Could you check a few things on this model? Use its own coordinates, in mm. Face numbers are marked on the shaded views. A direction names the side the tool comes from. Coordinates: 2 decimals unless noted, no trailing zeros. Loops run counter-clockwise (first coordinate to the right, second up) from the corner with the lowest first, then second, coordinate; pieces in that order, holes last.
1) If I drill on line 1 along Y through (x, z) = (51.65, 24.1); line 2 along X through (y, z) = (0.2, 13.5); line 3 along Z through (x, y) = (21.5, 35), over which ranges is the centre line in solid material (lowest first)?
2) Imagine slicing it at B-B on y = 40.25. Please give me the cut outline in (x, z), plus the area to 3 significant figures.
3) Imagine slicing it at D-D on x = 51.65. Please give me the cut outline in (y, z).
4) Imagine slicing it at C-C on z = 13.5. Please give me the cut outline in (x, y), plus the area to 3 significant figures.
5) Will these pins go through, and if not, where does the flat tip stop? P1, Ø3, axis at x = 20.65, y = 40.25, coming from the +Z side (3 decimals); P2, Ø3, axis at y = 34, z = 22, coming from the -X side; P3, Ø9, axis at x = 64.8, z = 13.5, coming from the +Y side; P4, Ø5.5, axis at x = 51.65, y = 9.25, coming from the -Z side.
6) For the marked faces 1 and 2, which set-ups out of +Z, -Z, +X, -X, +Y, -Y let a thin tool reach every point of the face, with its end or its side?
7) Imagine slicing it at A-A on x = 7.5. Please give me the cut outline in (y, z).
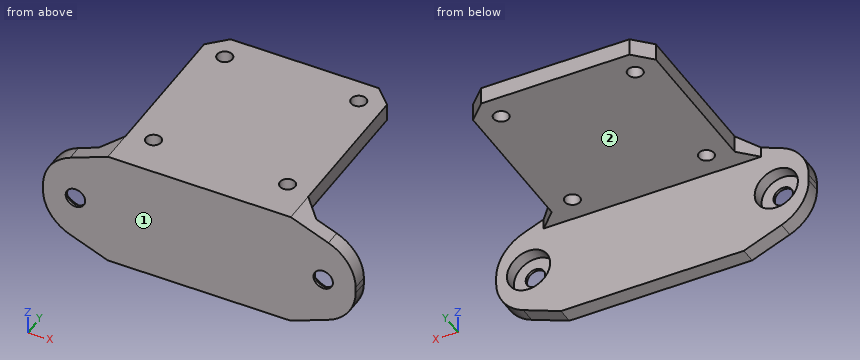
```python
from build123d import *

# Parameters (mm, degrees)
SCHIZZO2_W                                           = 72.3
SCHIZZO2_H                                           = 27
ESTRUSIONE_ESTRUSIONE1_DEPTH                         = 3.6
SCHIZZO3_W                                           = 42.3
SCHIZZO3_H                                           = 4
ESTRUSIONE_ESTRUSIONE2_DEPTH                         = 42.3
SCHIZZO4_R                                           = 1.75
TAGLIO_ESTRUSIONE1_DEPTH                             = 42.3
FORO_LAMATO_PER_VITE_M4_A_TESTA_CILINDRI_D           = 4.5
FORO_LAMATO_PER_VITE_M4_A_TESTA_CILINDRI_DEPTH       = 9
FORO_LAMATO_PER_VITE_M4_A_TESTA_CILINDRI_CBORE_D     = 10
FORO_LAMATO_PER_VITE_M4_A_TESTA_CILINDRI_CBORE_DEPTH = 3
FORO_LAMATO_PER_VITE_M4_A_TESTA_CILINDRI_TIP         = 1.351936393
TAGLIO_ESTRUSIONE2_DEPTH                             = 42.3
SMUSSO1_SIZE                                         = 4
RACCORDO1_R                                          = 10
SMUSSO2_SIZE                                         = 4


with BuildPart() as part:
    # Schizzo2 → Estrusione-Estrusione1 (new body)
    with BuildSketch(Plane(origin=(0, 0, 0), x_dir=(1, 0, 0), z_dir=(0, 1, 0))):
        with Locations((36.15, -13.5)):
            Rectangle(SCHIZZO2_W, SCHIZZO2_H)
    extrude(amount=ESTRUSIONE_ESTRUSIONE1_DEPTH)

    # Schizzo3 → Estrusione-Estrusione2 (add)
    with BuildSketch(Plane(origin=(0, 3.6, 0), x_dir=(1, 0, 0), z_dir=(0, 1, 0))):
        with Locations((36.15, -25)):
            Rectangle(SCHIZZO3_W, SCHIZZO3_H)
    extrude(amount=ESTRUSIONE_ESTRUSIONE2_DEPTH)

    # Schizzo4 → Taglio-Estrusione1 (cut)
    with BuildSketch(Plane.XY.offset(27)):
        with Locations((20.65, 40.25)):
            Circle(SCHIZZO4_R)
        with Locations((51.65, 40.25)):
            Circle(SCHIZZO4_R)
        with Locations((51.65, 9.25)):
            Circle(SCHIZZO4_R)
        with Locations((20.65, 9.25)):
            Circle(SCHIZZO4_R)
    extrude(amount=-TAGLIO_ESTRUSIONE1_DEPTH, mode=Mode.SUBTRACT)

    # Foro lamato per Vite M4 a testa cilindrica-2
    with Locations(Plane(origin=(0, 3.6, 0), x_dir=(1, 0, 0), z_dir=(0, 1, 0))):
        with Locations((7.5, -13.5), (64.8, -13.5)):
            CounterBoreHole(FORO_LAMATO_PER_VITE_M4_A_TESTA_CILINDRI_D / 2, FORO_LAMATO_PER_VITE_M4_A_TESTA_CILINDRI_CBORE_D / 2, FORO_LAMATO_PER_VITE_M4_A_TESTA_CILINDRI_CBORE_DEPTH, depth=FORO_LAMATO_PER_VITE_M4_A_TESTA_CILINDRI_DEPTH)
            with Locations((0, 0, -(FORO_LAMATO_PER_VITE_M4_A_TESTA_CILINDRI_DEPTH + FORO_LAMATO_PER_VITE_M4_A_TESTA_CILINDRI_TIP / 2))):  # 118° drill point
                Cone(0, FORO_LAMATO_PER_VITE_M4_A_TESTA_CILINDRI_D / 2, FORO_LAMATO_PER_VITE_M4_A_TESTA_CILINDRI_TIP, mode=Mode.SUBTRACT)

    # Schizzo8 → Taglio-Estrusione2 (cut)
    with BuildSketch(Plane(origin=(0, 3.6, 0), x_dir=(1, 0, 0), z_dir=(0, 1, 0))):
        Polygon((15, -27), (0, -21), (0, -27), align=None)
        Polygon((0, -6), (0, 0), (15, 0), align=None)
        Polygon((57.3, 0), (72.3, 0), (72.3, -6), align=None)
        Polygon((57.3, -27), (72.3, -27), (72.3, -21), align=None)
    extrude(amount=-TAGLIO_ESTRUSIONE2_DEPTH, mode=Mode.SUBTRACT)

    # Smusso1
    smusso1_edges = [part.edges().sort_by_distance(p)[0] for p in [
        (15, 45.9, 25),
        (57.3, 45.9, 25),
    ]]
    chamfer(smusso1_edges, length=SMUSSO1_SIZE)

    # Raccordo1
    raccordo1_edges = [part.edges().sort_by_distance(p)[0] for p in [
        (0, 1.8, 21),
        (72.3, 1.8, 21),
        (72.3, 1.8, 6),
        (0, 1.8, 6),
    ]]
    fillet(raccordo1_edges, radius=RACCORDO1_R)

    # Smusso2
    smusso2_edges = [part.edges().sort_by_distance(p)[0] for p in [
        (15, 3.6, 25),
        (57.3, 3.6, 25),
    ]]
    chamfer(smusso2_edges, length=SMUSSO2_SIZE)


solid = part.part
```
Filled in:
1. line 1: y = 0 to 7.5, 11 to 38.5, 42 to 45.9
1. line 2: x = 0 to 5.25, 9.75 to 62.55, 67.05 to 72.3
1. line 3: z = 23 to 27
2. outline: (15, 23) - (18.9, 23) - (18.9, 27) - (15, 27) - close; (22.4, 23) - (49.9, 23) - (49.9, 27) - (22.4, 27) - close; (53.4, 23) - (57.3, 23) - (57.3, 27) - (53.4, 27) - close
2. area: 141 mm2
3. outline: (0, 0) - (3.6, 0) - (3.6, 23) - (7.5, 23) - (7.5, 27) - (0, 27) - close; (11, 23) - (38.5, 23) - (38.5, 27) - (11, 27) - close; (42, 23) - (45.9, 23) - (45.9, 27) - (42, 27) - close
4. outline: (0, 0) - (5.25, 0) - (5.25, 0.6) - (2.5, 0.6) - (2.5, 3.6) - (0, 3.6) - close; (9.75, 0) - (62.55, 0) - (62.55, 0.6) - (59.8, 0.6) - (59.8, 3.6) - (12.5, 3.6) - (12.5, 0.6) - (9.75, 0.6) - close; (67.05, 0) - (72.3, 0) - (72.3, 3.6) - (69.8, 3.6) - (69.8, 0.6) - (67.05, 0.6) - close
4. area: 195 mm2
5. P1: passes through
5. P2: stops at x = 15
5. P3: stops at y = 0.6
5. P4: stops at z = 23
6. face 1: +Z, -Z, +X, -X, -Y
6. face 2: -Z, +X, -X, +Y
7. outline: (0, 3) - (3.6, 3) - (3.6, 8.5) - (0.6, 8.5) - (0.6, 11.25) - (0, 11.25) - close; (0, 15.75) - (0.6, 15.75) - (0.6, 18.5) - (3.6, 18.5) - (3.6, 24) - (0, 24) - close
